Geometry: final body of the model. Coordinates: model frame, mm. Face numbers are marked on the shaded views. A direction names the side the tool comes from. Give positions to 0.01 mm unless a question says otherwise; leave off trailing zeros. Order: outer loops, then holes, each group sorted by start corner. A loop starts at its lowest first (then second) coordinate and runs counter-clockwise, first axis right, second up. Notation, with made-up numbers: (15, 38.25) - (61, 38.25) arc R26 cw to (61, 72.25) - close; hole circle Ø3 at (83, -0.5). An arc over 180 degrees is marked (long way). Use one line per item in the form item = value.
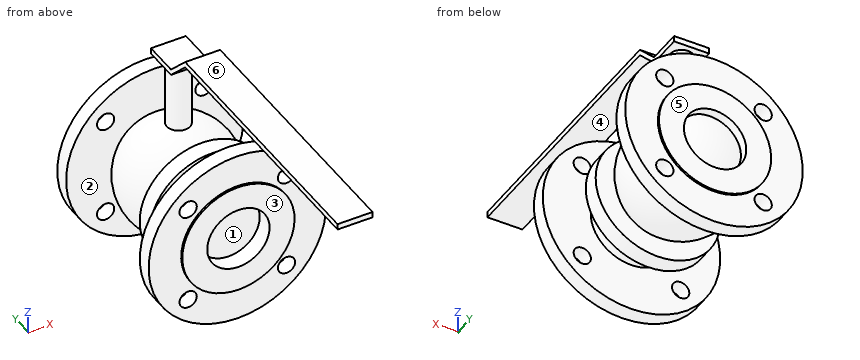
Autodesk Inventor part; units mm, degrees
ref_plane "Work Plane1" through (0, -36.75, 0) normal (0, -1, 0) x (1, 0, 0)
ref_plane "YZ Plane" through (0, 0, 0) normal (1, 0, 0) x (0, 1, 0)
ref_plane "XZ Plane" through (0, 0, 0) normal (0, 1, 0) x (-1, 0, 0)
sketch "Sketch1" plane through (0, 0, 0) normal (1, 0, 0) x (0, 1, 0)
  line L0 (67, 32.5) -> (83, 32.5)
  line L1 (83, 32.5) -> (83, 92.5)
  line L2 (83, 92.5) -> (67, 92.5)
  line L3 (67, 92.5) -> (67, 32.5)
  line L4 (83, 32.5) -> (85, 32.5)
  line L5 (85, 32.5) -> (85, 58.5)
  line L6 (85, 58.5) -> (83, 58.5)
  line L7 (83, 58.5) -> (83, 32.5)
  line L8 (-85, 0) -> (85, 0) construction
  line L9 (85, 0) -> (67, 0) construction
  line L10 (0, 0) -> (0, 98.124) construction
  line L11 (-85, 0) -> (-67, 0) construction
  line L12 (0, 0) -> (-17.7833, 0)
  dimension "Lenght" = 170
  dimension "DN" = 65
  dimension "FlgDia" = 185
  dimension "FlgThck" = 18
  dimension "GsktFace" = 117
  dimension "Face" = 2
revolve "Revolution1" add sketch "Sketch1" angle 360 about axis through (0, -85, 0) along (0, 1, 0)
sketch "Sketch5" plane through (0, 83, 0) normal (0, 1, 0) x (1, 0, 0)
  line L0 (0, 0) -> (-51.2652, 51.2652)
  line L1 (0, 0) -> (0, 103.939) construction
  circle A0 centre (-51.2652, 51.2652) radius 9
  point P0 (0, 0)
  dimension "d16" = 72.5
  dimension "d17" = 45
  dimension "d18" = 18
extrude "Extrusion2" cut sketch "Sketch5" against normal through all
pattern_circular "Circular Pattern1" count 4 over 360 about axis through (0, 84, 0) along (0, 1, 0) of "Extrusion2"
sketch "Sketch14" plane through (0, 67, 0) normal (0, -1, 0) x (-1, 0, 0)
  circle A0 centre (0, 0) radius 32.5
  circle A1 centre (0, 0) radius 42.5
  dimension "d54" = 10
pattern_circular "Circular Pattern2" count 2 over 360 about axis through (-10, 0, 0) along (1, 0, 0) of "Revolution1", "Extrusion2", "Circular Pattern1"
extrude "Extrusion5" add sketch "Sketch14" along normal up to surface (134 mm away) contours A0 | A1
sketch "Sketch20" plane through (0, 0, 0) normal (1, 0, 0) x (0, 1, 0)
  line L0 (24, -60.75) -> (24, 60.75)
  arc A0 (24, -60.75) -> (24, 60.75) centre (24, 0) ccw
  line L1 (85, -67.3299) -> (85, 28.8182)
  line L2 (24, 0) -> (36.15, 0)
  line L3 (36.15, 0) -> (36.15, 133)
  line L4 (36.15, 133) -> (24, 133)
  line L5 (24, 133) -> (24, 0)
  line L6 (42.225, 133) -> (5.775, 133)
  line L7 (5.775, 133) -> (5.775, 139.075)
  line L8 (5.775, 139.075) -> (42.225, 139.075)
  line L9 (42.225, 139.075) -> (42.225, 133)
  line L10 (-19.999, 164.849) -> (-297, 164.849)
  line L11 (-297, 164.849) -> (-297, 158.774)
  line L12 (-297, 158.774) -> (-19.999, 158.774)
  line L13 (-19.999, 158.774) -> (-19.999, 164.849)
  line L14 (-19.999, 158.774) -> (5.775, 133)
  line L15 (5.775, 139.075) -> (-19.999, 164.849)
  line L16 (67, -42.5) -> (67, 42.5)
  line L17 (-67, 42.5) -> (-67, -42.5)
  line L18 (85, -32.5) -> (85, 32.5)
  line L19 (85, -58.5) -> (85, 58.5)
  point P0 (0, 0)
  point P1 (24, -8.4077)
  point P2 (24, -8.4077)
  point P3 (85, -67.3299)
  point P4 (85, 28.8182)
  dimension "d78" = 121.5
  dimension "oI" = 61
  dimension "oH" = 133
  dimension "d81" = 12.15
  dimension "d85" = 135
  dimension "d86" = 6.075
  dimension "d87" = 6.075
  dimension "oW" = 321
  dimension "d89" = 36.45
revolve "Revolution5" add sketch "Sketch20" angle 360 about axis through (0, 24, 133) along (0, 0, -1) contours L0 L2 L3 A0 | L0 A0 L3 L2 | A0 L5 L4 L3
extrude "Extrusion8" add sketch "Sketch20" along normal mid plane 36.45 contours L4 L6 L7 L8 L9 | L14 L13 L15 L7 | L12 L11 L10 L13
ref_plane "Work Plane1" through (0, -36.75, 0) normal (0, -1, 0) x (1, 0, 0)
sketch "Sketch21" plane through (0, -36.75, 0) normal (0, -1, 0) x (1, 0, 0)
  circle A0 centre (0, 0) radius 42.5
  circle A1 centre (0, 0) radius 65
  point P0 (0, 0)
  dimension "d92" = 130
extrude "Extrusion9" add sketch "Sketch21" against normal blind 18
equation "\"d16\" = 0.5 * KDia"
equation "\"KDia\" = 145"
properties part number "BALL VALVE FLANGED DN65" material "S235"
(1) Pull-direction query (Z, two-part tool) for the marked faces 4, 5 and 6; classes: released by +Z, released by -Z, zero draft, split by the parting line, or undercut.
Computed values:
face_4 = undercut
face_5 = zero draft
face_6 = released by +Z
(2) Cut plane B-B on y = 24. Output: boundary loops of the cut face in (x, z) (3 decimals), plus the area to 3 significant figures.
Computed values:
outline = (-18.225, 133) - (-12.15, 133) - (-12.15, 59.523) arc R60.75 ccw (long way) to (12.15, 59.523) - (12.15, 133) - (18.225, 133) - (18.225, 139.075) - (-18.225, 139.075) - close
area = 13,600 mm²
(3) Cut plane C-C on y = -132. Output: boundary loops of the cut face in (x, z) (3 decimals).
Computed values:
outline = (-18.225, 158.774) - (18.225, 158.774) - (18.225, 164.849) - (-18.225, 164.849) - close
(4) Reachability of the marked faces 1, 2 and 3 from +Z, -Z, +X, -X, +Y, -Y: full face, straight path, thin tool, end or side. Return the list, or none.
Computed values:
face_1 = -Y
face_2 = none
face_3 = -Z, +X, -X, -Y
(5) Contact query for flat-ended pins moving along their axis: pin 1 Ø16 at (x, z) = (-51.27, -51.27) entering from -Y; pin 2 Ø20.5 at (x, z) = (-51.27, 51.27) entering from -Y; pin 3 Ø8 at (x, y) = (15.5, -14.5) entering from +Z. Output: stop coordinate, or through.
Computed values:
pin_1 = -36.75
pin_2 = -83
pin_3 = 163.35
(6) Ray query, line 1 along Z through (x, y) = (4.5, -73.5); line 2 along Y through (x, z) = (-6.5, 82.5); line 3 along Y through (x, z) = (34, 43.5). Return the intervals inside material, ascending.
Computed values:
line_1 = -92.39 to -32.19, 32.19 to 92.39, 158.77 to 164.85
line_2 = -83 to -67, 13.73 to 34.27, 67 to 83
line_3 = -85 to -67, -36.75 to -18.75, -1.34 to 49.34, 67 to 85
(7) Cut plane A-A on y = -48.5. Output: boundary loops of the cut face in (x, z) (3 decimals), plus the area to 3 significant figures.
Computed values:
outline = circle Ø85 at (0, 0); (-18.225, 158.774) - (18.225, 158.774) - (18.225, 164.849) - (-18.225, 164.849) - close
area = 5,900 mm²
